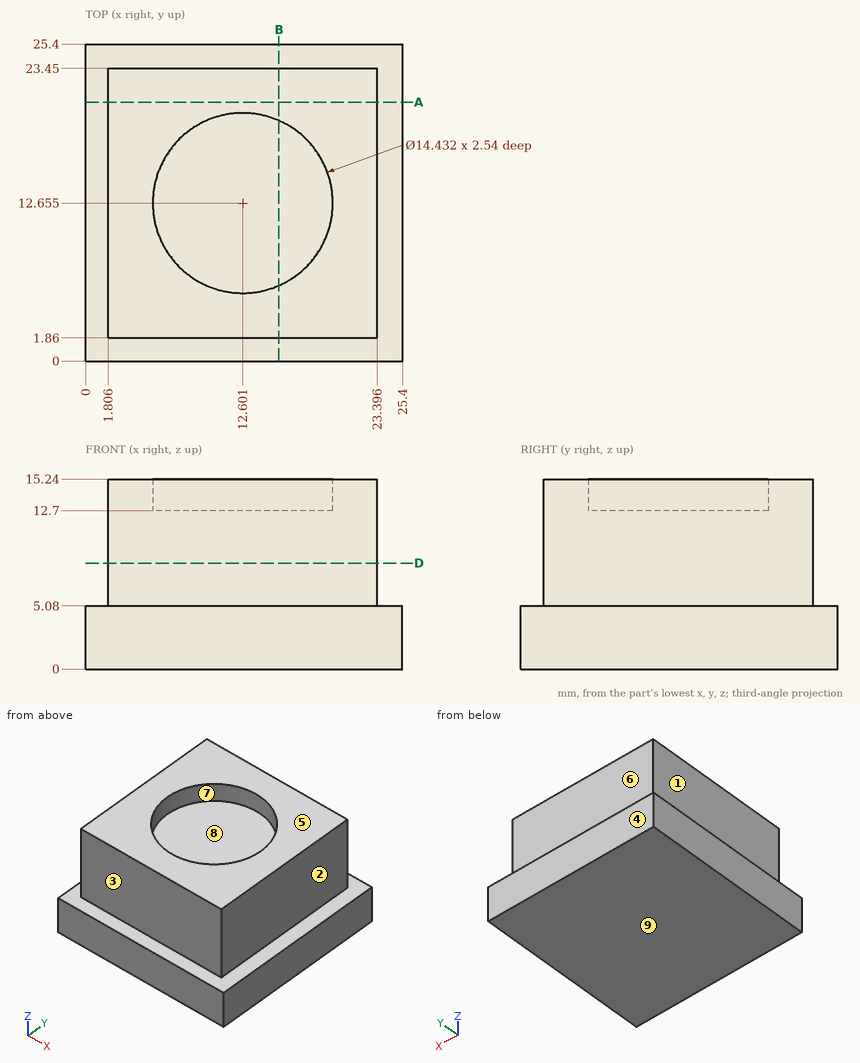
The figure shows three views and two pictorial views of one solid part (mm, origin at its lowest corner). Answer the questions. A direction names the side the tool comes from. Round coordinates to 2 decimals unless told otherwise and drop trailing zeros. Order: outer loops, then holes, each group sorted by start corner. A loop starts at its lowest first (then second) coordinate and runs counter-clockwise, first axis right, second up. Notation, with made-up numbers: M 35.25,16.5 L 46.25,16.5 A4 ccw 46.25,20.5 Z; hole C 63,-14.5 d8. An arc over 180 degrees is marked long. Put each result on its own line as item: value. Start each with the question number.
Q1. Straight lines are drawn through the part: L1, parallel to Y at x = 7.5, z = 11.5; L2, parallel to X at y = 11.5, z = 7.25; L3, parallel to Z at x = 10, y = 10. For each, find the intervals that lie inside material, in ascending order. Write a range as [from, to].
Q2. Section B-B, the plane x = 15.5 is taken. Write down the section's boundary in (y, z), and give its area (3 significant figures).
Q3. Section D-D, the plane z = 8.5 is taken. Write down the section's boundary in (x, y), and give its area (3 significant figures).
Q4. Section A-A, the plane y = 20.75 is taken. Write down the section's boundary in (x, z).
Q5. A tool of negligible diameter and unlimited length cuts with its end or side. For the marked faces 1, 2, 3, 4 and 5, from which of +Z, -Z, +X, -X, +Y, -Y can it reach the whole face along a straight path? Write none if from no direction.
Q6. Flat-ended cylindrical pins translate along their axes: pin 1 (8 mm diameter, centred on y = 16.5, z = 12, fed in from -X); pin 2 (1.5 mm diameter, centred on x = 13, z = 10.5, fed in from +Y); pin 3 (8 mm diameter, centred on y = 17.5, z = 10.5, fed in from +X). Find the tip coordinate at first contact, or state that the pin passes through.
Q7. For a pull along Y with two mould halves and no side action, classify the marked faces 6, 7, 8 and 9 as pulls with the +Y half, pulls with the -Y half, needs draft (parallel to the pull), parting line crosses it, or undercut.
Findings below:
1. L1: y = [1.86, 23.45]
1. L2: x = [1.81, 23.4]
1. L3: z = [0, 12.7]
2. outline: M 0,0 L 25.4,0 L 25.4,5.08 L 23.45,5.08 L 23.45,15.24 L 19.26,15.24 L 19.26,12.7 L 6.05,12.7 L 6.05,15.24 L 1.86,15.24 L 1.86,5.08 L 0,5.08 Z
2. area: 315 mm^2
3. outline: M 1.81,1.86 L 23.4,1.86 L 23.4,23.45 L 1.81,23.45 Z
3. area: 466 mm^2
4. outline: M 0,0 L 25.4,0 L 25.4,5.08 L 23.4,5.08 L 23.4,15.24 L 1.81,15.24 L 1.81,5.08 L 0,5.08 Z
5. face 1: +Z, -X, +Y, -Y
5. face 2: +Z, +X, +Y, -Y
5. face 3: +Z, +X, -X, -Y
5. face 4: +Z, -Z, +X, -X, +Y
5. face 5: +Z, +X, -X, +Y, -Y
6. pin 1: stops at x = 1.81
6. pin 2: stops at y = 23.45
6. pin 3: stops at x = 23.4
7. face 6: pulls with the +Y half
7. face 7: undercut
7. face 8: undercut
7. face 9: needs draft
